from build123d import *

# Parameters (mm, degrees)
F1_DEPTH  = 22
F2_T      = -2.5
F3_R      = 3
F3_R_2    = 1.4999993145
F4_DEPTH  = 19.5
F6_DEPTH  = 2.5
F7_W      = 9
F7_H      = 5
F8_DEPTH  = 2.5
F9_R      = 2.5
F9_R_2    = 1.5
F10_DEPTH = 10.5


with BuildPart() as f1:
    # F0 (on Top) → F1 (new body)
    with BuildSketch(Plane.XY):
        with BuildLine():
            ThreePointArc((42.5, 20.5), (41.6213203436, 22.6213203436), (39.5, 23.5))
            Line((39.5, 23.5), (-39.5, 23.5))
            ThreePointArc((-39.5, 23.5), (-41.6213203436, 22.6213203436), (-42.5, 20.5))
            Line((-42.5, 20.5), (-42.5, -20.5))
            ThreePointArc((-42.5, -20.5), (-41.6213203436, -22.6213203436), (-39.5, -23.5))
            Line((-39.5, -23.5), (39.5, -23.5))
            ThreePointArc((39.5, -23.5), (41.6213203436, -22.6213203436), (42.5, -20.5))
            Line((42.5, -20.5), (42.5, 20.5))
        make_face()
    extrude(amount=F1_DEPTH)

    # F2
    f2_openings = [f1.faces().sort_by_distance(p)[0] for p in [
        (0, 0, 22),
    ]]
    offset(amount=F2_T, openings=f2_openings)

    # F3 (on face) → F4 (join, through all)
    with BuildSketch(Plane.XY.offset(2.5)):
        with Locations((-38, 19)):
            Circle(F3_R)
        with Locations((-38, 19)):
            Circle(F3_R_2, mode=Mode.SUBTRACT)
        with Locations((38, 19)):
            Circle(F3_R)
        with Locations((38, 19)):
            Circle(F3_R_2, mode=Mode.SUBTRACT)
        with Locations((38, -19)):
            Circle(F3_R)
        with Locations((38, -19)):
            Circle(F3_R_2, mode=Mode.SUBTRACT)
        with Locations((-38, -19)):
            Circle(F3_R)
        with Locations((-38, -19)):
            Circle(F3_R_2, mode=Mode.SUBTRACT)
    extrude(amount=F4_DEPTH)

    # F5 (on face) → F6 (cut, through all)
    with BuildSketch(Plane.YZ.offset(42.5)):
        Polygon((7, 15), (-12, 15), (-12, 8), (-4.5, 8), (-4.5, 6.7), (-0.5, 6.7), (-0.5, 8), (7, 8), align=None)
    extrude(amount=-F6_DEPTH, mode=Mode.SUBTRACT)

    # F7 (on face) → F8 (cut, through all)
    with BuildSketch(Plane(origin=(0, 23.5, 0), x_dir=(-1, 0, 0), z_dir=(0, 1, 0))):
        with Locations((-19, 9.5)):
            Rectangle(F7_W, F7_H)
    extrude(amount=-F8_DEPTH, mode=Mode.SUBTRACT)

    # F9 (on face) → F10 (join)
    with BuildSketch(Plane.XY.offset(2.5)):
        with Locations((30, 14)):
            Circle(F9_R)
        with Locations((30, 14)):
            Circle(F9_R_2, mode=Mode.SUBTRACT)
        with Locations((30, -14)):
            Circle(F9_R)
        with Locations((30, -14)):
            Circle(F9_R_2, mode=Mode.SUBTRACT)
    extrude(amount=F10_DEPTH)


solid = f1.part
Check sheet for the modelled part. Datum: model origin and axes. Units: mm. A direction names the side the tool comes from. Coordinates: 2 decimals unless noted, no trailing zeros. Loops run counter-clockwise (first coordinate to the right, second up) from the corner with the lowest first, then second, coordinate; pieces in that order, holes last. Notation, with made-up numbers: (18.25, 35) -> (25.25, 35) arc R28 ccw to (25.25, 53) -> close; hole circle Ø1 at (83.25, 57). An arc over 180 degrees is marked (long way). Answer in a Markdown table with one row per item.
1. Sectioned sample at D-D, the plane y = 19. Record the boundary of the cut face in (x, z).
Check values:
| item | result |
|---|---|
| outline | (-42.5, 0) -> (42.5, 0) -> (42.5, 22) -> (39.5, 22) -> (39.5, 2.5) -> (36.5, 2.5) -> (36.5, 22) -> (35, 22) -> (35, 2.5) -> (-35, 2.5) -> (-35, 22) -> (-36.5, 22) -> (-36.5, 2.5) -> (-39.5, 2.5) -> (-39.5, 22) -> (-42.5, 22) -> close |
2. Sectioned sample at C-C, the plane x = 22. Record the boundary of the cut face in (y, z), then the cut area to 4 significant figures.
Check values:
| item | result |
|---|---|
| outline | (-23.5, 0) -> (23.5, 0) -> (23.5, 7) -> (21, 7) -> (21, 2.5) -> (-21, 2.5) -> (-21, 22) -> (-23.5, 22) -> close; (21, 12) -> (23.5, 12) -> (23.5, 22) -> (21, 22) -> close |
| area | 202.5 mm2 |
3. Sectioned sample at B-B, the plane y = -10. Record the boundary of the cut face in (x, z), then the cut area to 4 significant figures.
Check values:
| item | result |
|---|---|
| outline | (-42.5, 0) -> (42.5, 0) -> (42.5, 8) -> (40, 8) -> (40, 2.5) -> (-40, 2.5) -> (-40, 22) -> (-42.5, 22) -> close; (40, 15) -> (42.5, 15) -> (42.5, 22) -> (40, 22) -> close |
| area | 292.5 mm2 |
4. Release check for a two-part mould opening along X. For faces 1 (the face through (35.924, -16.834, 12.114)), 2 (the face through (42.5, 0, 6)), 3 (the face through (41, -2, 15)) record: released by +X, released by -X, zero draft, split by the parting line, or undercut.
Check values:
| item | result |
|---|---|
| face 1 | undercut |
| face 2 | released by +X |
| face 3 | zero draft |
5. Material ranges on line 1 along Y through (x, z) = (30, 5.5); line 2 along Y through (x, z) = (32, 4.5); line 3 along Y through (x, z) = (33, 10.5), recorded low to high. Write a range as [from, to].
Check values:
| item | result |
|---|---|
| line 1 | y = [-23.5, -21], [-16.5, -15.5], [-12.5, -11.5], [11.5, 12.5], [15.5, 16.5], [21, 23.5] |
| line 2 | y = [-23.5, -21], [-15.5, -12.5], [12.5, 15.5], [21, 23.5] |
| line 3 | y = [-23.5, -21], [21, 23.5] |
6. Access from +Z, -Z, +X, -X, +Y, -Y to the whole of each face (thin tool, end or side, straight path). Record for faces 4 (the face through (41.6, -22.64, 10.85)), 5 (the face through (-1, 0, 0)), 6 (the face through (1, 21, 12)), 7 (the face through (41, -12, 12)), 8 (the face through (19, 22, 7)).
Check values:
| item | result |
|---|---|
| face 4 | +Z, -Z, +X, -Y |
| face 5 | -Z, +X, -X, +Y, -Y |
| face 6 | +Z |
| face 7 | +X |
| face 8 | +Y |
7. Sectioned sample at A-A, the plane z = 5.75. Give the number of separate pieces and of enclosed holes in the cut face, then the cut area to 3 significant figures.
Check values:
| item | result |
|---|---|
| separate pieces | 3 |
| enclosed holes | 7 |
| area | 713 mm2 |
8. Go/stop test with flat-tipped pins: pin 1 (6 mm diameter, centred on x = -12.5, y = -2.5, fed in from +Z); pin 2 (1 mm diameter, centred on x = 41.5, z = 7.5, fed in from +Y); pin 3 (3.5 mm diameter, centred on x = 30, y = -14, fed in from +Z). Record where each tip stops, or that it passes through.
Check values:
| item | result |
|---|---|
| pin 1 | stops at z = 2.5 |
| pin 2 | stops at y = 23.1 |
| pin 3 | stops at z = 13 |
